Can you work these out from the model? Positions are in its coordinate system, mm. Face numbers are marked on the shaded views. A direction names the side the tool comes from. Give positions to 0.01 mm unless a question says otherwise; leave off trailing zeros. Loops run counter-clockwise (first coordinate to the right, second up) from the corner with the lowest first, then second, coordinate; pieces in that order, holes last. Notation, with made-up numbers: (-8.5, 48) - (46.5, 48) arc R23 cw to (46.5, 77) - close; hole circle Ø7 at (88.5, -14.5). An arc over 180 degrees is marked (long way). Answer in a Markdown table with one row per item.
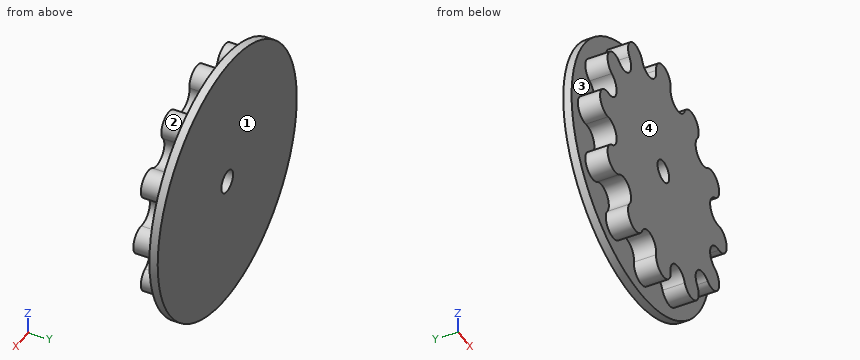
from build123d import *

# Parameters (mm, degrees)
BOSS_EXTRUDE1_DEPTH = 8
SKETCH3_R           = 47.5
BOSS_EXTRUDE2_DEPTH = 3
SKETCH4_R           = 4
CUT_EXTRUDE1_DEPTH  = 30


with BuildPart() as part:
    # Sketch1 → Boss-Extrude1 (new body)
    with BuildSketch(Plane(origin=(0, 0, 0), x_dir=(1, 0, 0), z_dir=(0, 1, 0))):
        with BuildLine():
            ThreePointArc((37.867444544, -4.985343651), (43.25, 0), (37.867444544, 4.985343651))
            ThreePointArc((37.867444544, 4.985343651), (32.117033724, 8.60573325), (35.286840777, 14.616288023))
            ThreePointArc((35.286840777, 14.616288023), (37.455598714, 21.625), (30.301497126, 23.251156521))
            ThreePointArc((30.301497126, 23.251156521), (23.511300474, 23.511300474), (23.251156521, 30.301497126))
            ThreePointArc((23.251156521, 30.301497126), (21.625, 37.455598714), (14.616288023, 35.286840777))
            ThreePointArc((14.616288023, 35.286840777), (8.60573325, 32.117033724), (4.985343651, 37.867444544))
            ThreePointArc((4.985343651, 37.867444544), (0, 43.25), (-4.985343651, 37.867444544))
            ThreePointArc((-4.985343651, 37.867444544), (-8.60573325, 32.117033724), (-14.616288023, 35.286840777))
            ThreePointArc((-14.616288023, 35.286840777), (-21.625, 37.455598714), (-23.251156521, 30.301497126))
            ThreePointArc((-23.251156521, 30.301497126), (-23.511300474, 23.511300474), (-30.301497126, 23.251156521))
            ThreePointArc((-30.301497126, 23.251156521), (-37.455598714, 21.625), (-35.286840777, 14.616288023))
            ThreePointArc((-35.286840777, 14.616288023), (-32.117033724, 8.60573325), (-37.867444544, 4.985343651))
            ThreePointArc((-37.867444544, 4.985343651), (-43.25, 0), (-37.867444544, -4.985343651))
            ThreePointArc((-37.867444544, -4.985343651), (-32.117033724, -8.60573325), (-35.286840777, -14.616288023))
            ThreePointArc((-35.286840777, -14.616288023), (-37.455598714, -21.625), (-30.301497126, -23.251156521))
            ThreePointArc((-30.301497126, -23.251156521), (-23.511300474, -23.511300474), (-23.251156521, -30.301497126))
            ThreePointArc((-23.251156521, -30.301497126), (-21.625, -37.455598714), (-14.616288023, -35.286840777))
            ThreePointArc((-14.616288023, -35.286840777), (-8.60573325, -32.117033724), (-4.985343651, -37.867444544))
            ThreePointArc((-4.985343651, -37.867444544), (0, -43.25), (4.985343651, -37.867444544))
            ThreePointArc((4.985343651, -37.867444544), (8.60573325, -32.117033724), (14.616288023, -35.286840777))
            ThreePointArc((14.616288023, -35.286840777), (21.625, -37.455598714), (23.251156521, -30.301497126))
            ThreePointArc((23.251156521, -30.301497126), (23.511300474, -23.511300474), (30.301497126, -23.251156521))
            ThreePointArc((30.301497126, -23.251156521), (37.455598714, -21.625), (35.286840777, -14.616288023))
            ThreePointArc((35.286840777, -14.616288023), (32.117033724, -8.60573325), (37.867444544, -4.985343651))
        make_face()
    extrude(amount=BOSS_EXTRUDE1_DEPTH)

    # Sketch3 → Boss-Extrude2 (add)
    with BuildSketch(Plane(origin=(0, 8, 0), x_dir=(1, 0, 0), z_dir=(0, 1, 0))):
        Circle(SKETCH3_R)
    extrude(amount=BOSS_EXTRUDE2_DEPTH)

    # Sketch4 → Cut-Extrude1 (cut)
    with BuildSketch(Plane(origin=(0, 11, 0), x_dir=(1, 0, 0), z_dir=(0, 1, 0))):
        Circle(SKETCH4_R)
    extrude(amount=-CUT_EXTRUDE1_DEPTH, mode=Mode.SUBTRACT)


solid = part.part
Q1. Imagine slicing it at B-B, the plane z = 0. Write out the boundary of the cut face in (x, y), and give its area (3 significant figures).
Checked values:
| item | result |
|---|---|
| outline | (-47.5, 8) - (-43.25, 8) - (-43.25, 0) - (-4, 0) - (-4, 11) - (-47.5, 11) - close; (4, 0) - (43.25, 0) - (43.25, 8) - (47.5, 8) - (47.5, 11) - (4, 11) - close |
| area | 889 mm² |
Q2. For pin 1 (1.5 mm diameter, centred on y = 3.5, z = 35, fed in from -X); pin 2 (1.5 mm diameter, centred on x = -14, y = 6.5, fed in from +Z); pin 3 (3 mm diameter, centred on x = 35.5, y = 1.5, fed in from +Z), each with a flat end and sliding along its axis, tell me the tip position at first contact or that it passes through.
Checked values:
| item | result |
|---|---|
| pin 1 | stops at x = -24 |
| pin 2 | stops at z = 35.55 |
| pin 3 | stops at z = 24.05 |
Q3. If we mould it in two halves opening along Z, with no side actions, what happens to the marked faces 1 and 2? For each: released by +Z, released by -Z, zero draft, split by the parting line, or undercut.
Checked values:
| item | result |
|---|---|
| face 1 | zero draft |
| face 2 | undercut |
Q4. If I drill on line 1 (X direction, y = 3, z = 34); line 2 (Y direction, x = 6, z = 40.5); line 3 (Z direction, x = 0, y = 8.75), over which ranges is the centre line in solid material (lowest first)? Write a range as [from, to].
Checked values:
| item | result |
|---|---|
| line 1 | x = [-24.05, -13.94], [-5.86, 5.86], [13.94, 24.05] |
| line 2 | y = [8, 11] |
| line 3 | z = [-47.5, -4], [4, 47.5] |
Q5. Imagine slicing it at A-A, the plane x = 0. Write out the boundary of the cut face in (y, z), and give its area (3 significant figures).
Checked values:
| item | result |
|---|---|
| outline | (0, -43.25) - (8, -43.25) - (8, -47.5) - (11, -47.5) - (11, -4) - (0, -4) - close; (0, 4) - (11, 4) - (11, 47.5) - (8, 47.5) - (8, 43.25) - (0, 43.25) - close |
| area | 889 mm² |
Q6. On a 3-axis mill with a long thin cutter (end or side, diameter ignored), from which of +Z, -Z, +X, -X, +Y, -Y can I reach the whole of each face in a straight line? I mean the marked faces 3 and 4. Say none if no direction works.
Checked values:
| item | result |
|---|---|
| face 3 | -Y |
| face 4 | +Z, -Z, +X, -X, -Y |
Q7. Imagine slicing it at D-D, the plane z = -19.5. Write out the boundary of the cut face in (x, y), and give its area (3 significant figures).
Checked values:
| item | result |
|---|---|
| outline | (-43.31, 8) - (-38.11, 8) - (-38.11, 0) - (38.11, 0) - (38.11, 8) - (43.31, 8) - (43.31, 11) - (-43.31, 11) - close |
| area | 870 mm² |
